from build123d import *

# Parameters (mm, degrees)
SKETCH_3_R      = 1.5
SKETCH_3_R_2    = 2
SKETCH_3_W      = 7.2
SKETCH_3_H      = 2.2
EXTRUDE_1_DEPTH = 2


with BuildPart() as part:
    # 草图3 → 凸台-拉伸1 (new body)
    with BuildSketch(Plane.XY):
        with BuildLine():
            Line((-46.5, 0.009783315), (-46.5, -3.990216685))
            Line((-46.5, -3.990216685), (-26.5, -3.990216685))
            Line((-26.5, -3.990216685), (-26.5, 3.009783315))
            Line((-26.5, 3.009783315), (26.5, 3.009783315))
            Line((26.5, 3.009783315), (26.5, -3.990216685))
            Line((26.5, -3.990216685), (46.5, -3.990216685))
            Line((46.5, -3.990216685), (46.5, 0.009783315))
            Line((46.5, 0.009783315), (49.5, 0.009783315))
            Line((49.5, 0.009783315), (49.5, 5.009783315))
            Line((49.5, 5.009783315), (46.5, 5.009783315))
            Line((46.5, 5.009783315), (46.5, 7.009783315))
            Line((46.5, 7.009783315), (44, 7.009783315))
            Line((44, 7.009783315), (44, 5.509783315))
            Line((44, 5.509783315), (41.4, 5.509783315))
            Line((41.4, 5.509783315), (41.4, 7.009783315))
            Line((41.4, 7.009783315), (38.4, 7.009783315))
            Line((38.4, 7.009783315), (38.4, 10.009783315))
            Line((38.4, 10.009783315), (41.4, 10.009783315))
            Line((41.4, 10.009783315), (41.4, 11.509783315))
            Line((41.4, 11.509783315), (44, 11.509783315))
            Line((44, 11.509783315), (44, 10.009783315))
            Line((44, 10.009783315), (46.5, 10.009783315))
            Line((46.5, 10.009783315), (46.5, 15.009783315))
            Line((46.5, 15.009783315), (49.5, 15.009783315))
            Line((49.5, 15.009783315), (49.5, 20.009783315))
            Line((49.5, 20.009783315), (46.5, 20.009783315))
            Line((46.5, 20.009783315), (46.5, 30.009783315))
            Line((46.5, 30.009783315), (34.06116735, 36.162324196))
            ThreePointArc((34.06116735, 36.162324196), (-11.38853896, 16.756491321), (-37.576612526, 58.666477673))
            Line((-37.576612526, 58.666477673), (-46.5, 60.009783315))
            Line((-46.5, 60.009783315), (-46.5, 20.009783315))
            Line((-46.5, 20.009783315), (-49.5, 20.009783315))
            Line((-49.5, 20.009783315), (-49.5, 15.009783315))
            Line((-49.5, 15.009783315), (-46.5, 15.009783315))
            Line((-46.5, 15.009783315), (-46.5, 10.009783315))
            Line((-46.5, 10.009783315), (-44, 10.009783315))
            Line((-44, 10.009783315), (-44, 11.509783315))
            Line((-44, 11.509783315), (-41.4, 11.509783315))
            Line((-41.4, 11.509783315), (-41.4, 10.009783315))
            Line((-41.4, 10.009783315), (-38.4, 10.009783315))
            Line((-38.4, 10.009783315), (-38.4, 7.009783315))
            Line((-38.4, 7.009783315), (-41.4, 7.009783315))
            Line((-41.4, 7.009783315), (-41.4, 5.509783315))
            Line((-41.4, 5.509783315), (-44, 5.509783315))
            Line((-44, 5.509783315), (-44, 7.009783315))
            Line((-44, 7.009783315), (-46.5, 7.009783315))
            Line((-46.5, 7.009783315), (-46.5, 5.009783315))
            Line((-46.5, 5.009783315), (-49.5, 5.009783315))
            Line((-49.5, 5.009783315), (-49.5, 0.009783315))
            Line((-49.5, 0.009783315), (-46.5, 0.009783315))
        make_face()
        with Locations((-31.5, -0.990216685)):
            Circle(SKETCH_3_R, mode=Mode.SUBTRACT)
        with Locations((31.5, -0.990216685)):
            Circle(SKETCH_3_R, mode=Mode.SUBTRACT)
        with Locations((0, 10.509783315)):
            Circle(SKETCH_3_R_2, mode=Mode.SUBTRACT)
        with Locations((-30.0520382, 22.957745114)):
            Circle(SKETCH_3_R_2, mode=Mode.SUBTRACT)
        with Locations((-42.5, 53.009783315)):
            Circle(SKETCH_3_R_2, mode=Mode.SUBTRACT)
        with Locations((30.0520382, 22.957745114)):
            Circle(SKETCH_3_R_2, mode=Mode.SUBTRACT)
        with Locations((-39, -0.990216685)):
            Rectangle(SKETCH_3_W, SKETCH_3_H, mode=Mode.SUBTRACT)
        with Locations((39, -0.990216685)):
            Rectangle(SKETCH_3_W, SKETCH_3_H, mode=Mode.SUBTRACT)
    extrude(amount=EXTRUDE_1_DEPTH)


solid = part.part
For this review, take the finished solid that the model builds, in its own axes (mm). A direction names the side the tool comes from. Round coordinates to 2 decimals unless told otherwise and drop trailing zeros. Order: outer loops, then holes, each group sorted by start corner. A loop starts at its lowest first (then second) coordinate and runs counter-clockwise, first axis right, second up. Notation, with made-up numbers: (56.5, -10.5) -> (70.5, -10.5) arc R28 ccw to (70.5, 13.5) -> close; hole circle Ø8 at (61.5, -34.75). An arc over 180 degrees is marked (long way). Write item = value, one per line. Start each with the question number.
1) The part is to be moulded in two halves that separate along X. For faces 1 (the face through (46.5, 12, 1)), 2 (the face through (0, 3.01, 1)), 3 (the face through (-40, 10.01, 1)), say which applies: +X half, -X half, draft (parallel to the pull), parting line (faces both ways), or undercut.
2) Take a section at C-C on z = 0.9. Count the separate pieces of the cut face and the enclosed holes in it, plus the area to 3 significant figures.
3) To check wall thickness, follow line 1 (Y direction, x = -31.5, z = 1.5); line 2 (Y direction, x = 42.5, z = 1.05); line 3 (Y direction, x = -42.5, z = 1.05). State the ranges of each line that lie inside material, in increasing order. Write a range as from..to.
4) Take a section at A-A on x = 0. State the section outline as (y, z) points.
5) Insertion check: pin 1 (0.6 mm diameter, centred on y = 8.5, z = 1, fed in from -X); pin 2 (1 mm diameter, centred on x = 6.5, z = 0.5, fed in from +Y); pin 3 (4 mm diameter, centred on x = 1, y = 4.5, fed in from -Z). Each pin has a flat end and moves straight along its axis. Give the tip position at first contact, or say it passes through.
6) Take a section at B-B on y = 22. State the section outline as (x, z) points, plus the area to 3 significant figures.
7) Tool access review of faces 4 (the face through (-48, 15.01, 1)), 5 (the face through (46.5, 25, 1)), 6 (the face through (48, 5.01, 1)), 7 (the face through (39, 0.11, 1)), 8 (the face through (-48, 0.01, 1)): name each direction out of +Z, -Z, +X, -X, +Y, -Y from which nothing blocks a thin tool from reaching the whole face with its end or side.
8) Take a section at D-D on x = -25. State the section outline as (y, z) points, plus the area to 3 significant figures.
Verdict:
q1.face_1 = +X half
q1.face_2 = undercut
q1.face_3 = draft
q2.separate_pieces = 1
q2.enclosed_holes = 8
q2.area = 2,410 mm2
q3.line_1 = -3.99..-2.49, 0.51..21.58, 24.34..31.76
q3.line_2 = -3.99..-2.09, 0.11..5.51, 11.51..31.99
q3.line_3 = -3.99..-2.09, 0.11..5.51, 11.51..51.01, 55.01..59.41
q4.outline = (3.01, 0) -> (8.51, 0) -> (8.51, 2) -> (3.01, 2) -> close; (12.51, 0) -> (15.01, 0) -> (15.01, 2) -> (12.51, 2) -> close
q5.pin_1 = -38.4
q5.pin_2 = 15.66
q5.pin_3 = 0
q6.outline = (-46.5, 0) -> (-31.81, 0) -> (-31.81, 2) -> (-46.5, 2) -> close; (-28.3, 0) -> (-21.96, 0) -> (-21.96, 2) -> (-28.3, 2) -> close; (21.96, 0) -> (28.3, 0) -> (28.3, 2) -> (21.96, 2) -> close; (31.81, 0) -> (46.5, 0) -> (46.5, 2) -> (31.81, 2) -> close
q6.area = 84.1 mm2
q7.face_4 = +Z, -Z, -X
q7.face_5 = +Z, -Z, +X, +Y
q7.face_6 = +Z, -Z, +X
q7.face_7 = +Z, -Z
q7.face_8 = +Z, -Z, -X, -Y
q8.outline = (3.01, 0) -> (24.39, 0) -> (24.39, 2) -> (3.01, 2) -> close
q8.area = 42.8 mm2
